Source: CAD feature listing. Evaluate the final solid. Frame: model axes, mm. Face numbers are marked on the shaded views. A direction names the side the tool comes from. Coordinates: 2 decimals unless noted, no trailing zeros. Order: outer loops, then holes, each group sorted by start corner. A loop starts at its lowest first (then second) coordinate and runs counter-clockwise, first axis right, second up.
```python
from build123d import *

# Parameters (mm, degrees)
F1_DEPTH = 38.1
F2_W     = 12.7
F2_H     = 11.142593
F3_DEPTH = 6.35


with BuildPart() as f1:
    # F0 (on Front) → F1 (new body)
    with BuildSketch(Plane.XZ):
        Polygon((-25.4, 0), (0, 0), (0, 31.75), (-12.7, 31.75), (-12.7, 12.7), (-25.4, 12.7), align=None)
    extrude(amount=F1_DEPTH)

    # F2 (on face) → F3 (cut)
    with BuildSketch(Plane.XY.offset(31.75)):
        with Locations((-6.35, -19.344779)):
            Rectangle(F2_W, F2_H)
    extrude(amount=-F3_DEPTH, mode=Mode.SUBTRACT)


solid = f1.part
```
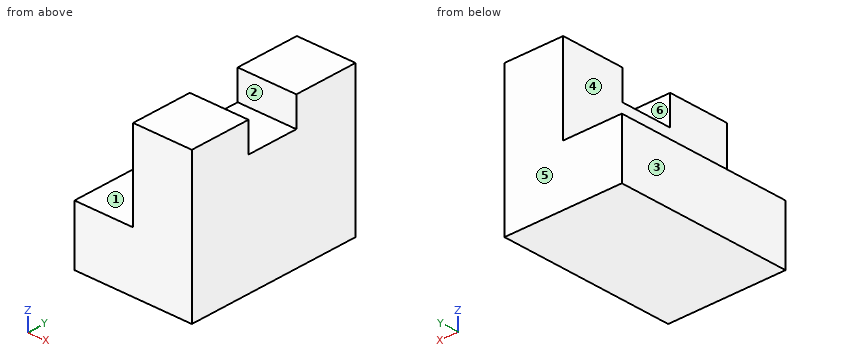
1. Access query for the marked faces 1, 2 and 3. Directions: +Z, -Z, +X, -X, +Y, -Y. A direction counts if a zero-diameter tool reaches every point of the face in a straight line with its end or side. Return the directions, or none.
Findings:
face 1: +Z, -X, +Y, -Y
face 2: +Z, +X, -X
face 3: +Z, -Z, -X, +Y, -Y
2. Section query C-C on y = -20. Return loops of the section in (x, z), plus the area to 3 significant figures.
Findings:
outline: (-25.4, 0) - (0, 0) - (0, 25.4) - (-12.7, 25.4) - (-12.7, 12.7) - (-25.4, 12.7) - close
area: 484 mm2
3. Section query D-D on z = 16. Return loops of the section in (x, y), plus the area to 3 significant figures.
Findings:
outline: (-12.7, -38.1) - (0, -38.1) - (0, 0) - (-12.7, 0) - close
area: 484 mm2
4. Pin query (flat end, axial travel): P1, Ø6, axis at x = -13, y = -17, coming from the +Z side; P2, Ø6.5, axis at x = -20.5, y = -27, coming from the +Z side. Return the tip coordinate at first contact, or that it passes through.
Findings:
P1: stops at z = 25.4
P2: stops at z = 12.7
5. Section query B-B on x = -2. Return loops of the section in (y, z).
Findings:
outline: (-38.1, 0) - (0, 0) - (0, 31.75) - (-13.77, 31.75) - (-13.77, 25.4) - (-24.92, 25.4) - (-24.92, 31.75) - (-38.1, 31.75) - close
6. Draft query along Y for the marked faces 4, 5 and 6. Return one class per face: released by +Y, released by -Y, zero draft, split by the parting line, or undercut.
Findings:
face 4: zero draft
face 5: released by +Y
face 6: undercut
7. Section query A-A on z = 29. Return loops of the section in (x, y).
Findings:
outline: (-12.7, -38.1) - (0, -38.1) - (0, -24.92) - (-12.7, -24.92) - close; (-12.7, -13.77) - (0, -13.77) - (0, 0) - (-12.7, 0) - close
8. Ray query, line 1 (Z direction, x = -17, y = -23.5); line 2 (Z direction, x = -3.75, y = -20); line 3 (X direction, y = -16.5, z = 13). Return the intervals inside material, ascending.
Findings:
line 1: z = 0 to 12.7
line 2: z = 0 to 25.4
line 3: x = -12.7 to 0
